Input: part model. Units: mm. Frame: model coordinates. A direction names the side the tool comes from. Give positions to 0.01 mm unless a question says otherwise; leave off trailing zeros. Order: outer loops, then holes, each group sorted by start corner. A loop starts at its lowest first (then second) coordinate and runs counter-clockwise, first axis right, second up. Notation, with made-up numbers: M 17,79 L 39,79 A27 ccw 39,114 Z; hole C -2.75,82 d6. An arc over 180 degrees is marked long. Use a Markdown table: item, result.
from build123d import *

# Parameters (mm, degrees)
F1_DEPTH = 982.5
F3_DEPTH = 50.001
F5_DEPTH = 8
F7_DEPTH = 8


with BuildPart() as f1:
    # F0 (on Top) → F1 (new body)
    with BuildSketch(Plane.XY):
        Polygon((0, 50), (0, 0), (50, 0), (50, 8), (8, 8), (8, 50), align=None)
    extrude(amount=F1_DEPTH)

    # F2 (on face) → F3 (cut, through all)
    with BuildSketch(Plane(origin=(0, 0, 0), x_dir=(0, -1, 0), z_dir=(-1, 0, 0))):
        Polygon((-50, 932.5), (0, 982.5), (-50, 982.5), align=None)
    extrude(amount=-F3_DEPTH, mode=Mode.SUBTRACT)

    # F4 (on face) → F5 (cut, through all)
    with BuildSketch(Plane.XZ):
        Polygon((50, 50), (0, 0), (50, 0), align=None)
    extrude(amount=-F5_DEPTH, mode=Mode.SUBTRACT)

    # F6 (on face) → F7 (cut, through all)
    with BuildSketch(Plane(origin=(0, 0, 0), x_dir=(0, -1, 0), z_dir=(-1, 0, 0))):
        Polygon((-8, 0), (0, 0), (-50, 50), (-50, 0), align=None)
    extrude(amount=-F7_DEPTH, mode=Mode.SUBTRACT)


solid = f1.part
1) Cut plane B-B on x = 41.5. Return loops of the section in (y, z).
Response values:
| item | result |
|---|---|
| outline | M 0,41.5 L 8,41.5 L 8,974.5 L 0,982.5 Z |
2) Cut plane C-C on y = 29. Return loops of the section in (x, z).
Response values:
| item | result |
|---|---|
| outline | M 0,29 L 8,29 L 8,953.5 L 0,953.5 Z |
3) Material intervals for line 1 (X direction, y = 35, z = 883.5); line 2 (Z direction, x = 31.5, y = 6.5), sorted ascending. Write a range as from..to.
Response values:
| item | result |
|---|---|
| line 1 | x = 0..8 |
| line 2 | z = 31.5..976 |
4) Cut plane A-A on z = 657.5. Return loops of the section in (x, y).
Response values:
| item | result |
|---|---|
| outline | M 0,0 L 50,0 L 50,8 L 8,8 L 8,50 L 0,50 Z |
5) First-contact query: pin 1 Ø10 at (x, z) = (17, 385.5) entering from +Y; pin 2 Ø5 at (y, z) = (23.5, 625) entering from +X. Flat tips, straight axial feed; report the tip coordinate or a pass-through.
Response values:
| item | result |
|---|---|
| pin 1 | stops at y = 8 |
| pin 2 | stops at x = 8 |
6) Reachability of faces 1 (the face through (29, 8, 484)), 2 (the face through (25, 0, 484)) from +Z, -Z, +X, -X, +Y, -Y: full face, straight path, thin tool, end or side. Return the list, or none.
Response values:
| item | result |
|---|---|
| face 1 | +Z, -Z, +X, +Y |
| face 2 | +Z, -Z, +X, -X, -Y |
